Build history of the part. All positions in model axes, mm. A direction names the side the tool comes from. Round coordinates to 2 decimals unless told otherwise and drop trailing zeros. Write each loop counter-clockwise with the first axis right and the second up, starting at its lowest first coordinate (ties: lowest second). Pieces come first, ordered by that corner, then holes. Notation, with made-up numbers: (-11, -26) -> (14, -26) arc R10 cw to (14, -22) -> close; hole circle Ø5 at (78.5, -10.75). An arc over 180 degrees is marked (long way). Answer in a Markdown table with one row per item. Add a question column.
from build123d import *

# Parameters (mm, degrees)
SKETCH1_W           = 20
SKETCH1_H           = 20
BOSS_EXTRUDE1_DEPTH = 10
SKETCH2_R           = 3


with BuildPart() as part:
    # Sketch1 → Boss-Extrude1 (new body)
    with BuildSketch(Plane(origin=(0, 0, 0), x_dir=(1, 0, 0), z_dir=(0, 1, 0))):
        Polygon((-59.044427996, 78.732050808), (-54.714300977, 76.232050808), (-38.661742094, 66.964101615), (-38.661742094, 85.5), (38.661742094, 85.5), (38.661742094, 66.964101615), (54.714300977, 76.232050808), (59.044427996, 78.732050808), (35.218366421, 120), (-35.218366421, 120), align=None)
        with Locations((0, 105)):
            Rectangle(SKETCH1_W, SKETCH1_H, mode=Mode.SUBTRACT)
    extrude(amount=BOSS_EXTRUDE1_DEPTH)

    # Cut-Sweep1: sweep along a path in Sketch3
    with BuildLine(Plane(origin=(0, 5, 0), x_dir=(1, 0, 0), z_dir=(0, 1, 0))) as cut_sweep1_path:
        Line((-38.661742094, 76), (-42.146569651, 76))
        ThreePointArc((-42.146569651, 76), (-43.646569651, 75.598076211), (-44.744645862, 74.5))
        Line((-44.744645862, 74.5), (-46.487059641, 71.482050808))
    # Sketch2 → Cut-Sweep1 (sweep, cut)
    with BuildSketch(Plane(origin=(-38.661742094, 0, 0), x_dir=(0, 0, -1), z_dir=(1, 0, 0))):
        with Locations((76, 5)):
            Circle(SKETCH2_R)
    cut_sweep1 = sweep(path=cut_sweep1_path.line, mode=Mode.SUBTRACT)

    # Mirror3: Cut-Sweep1 across plane
    add(cut_sweep1.mirror(Plane(origin=(0, 0, 0), x_dir=(0, 0, 1), z_dir=(1, 0, 0))), mode=Mode.SUBTRACT)


solid = part.part
(1) Saw through at D-D (z = -98). List the corners of the cut face in (x, y), plus the area to 3 significant figures.
(2) Saw through at A-A (y = 3.5). List the corners of the cut face in (x, z).
(3) Mould opens along Z. For faces 1 (the face through (-1, 5, -85.5)), 2 (the face through (48.106, 4.099, -74.401)), 3 (the face through (47.298, 4.93, -99.077)) say: pulls with the +Z half, pulls with the -Z half, needs draft (parallel to the pull), parting line crosses it, or undercut.
(4) Saw through at C-C (x = 11.5). List the corners of the cut face in (y, z), plus the area to 3 significant figures.
(5) Saw through at B-B (z = -105.5). List the corners of the cut face in (x, y), plus the area to 3 significant figures.
(6) Probe line 1 along Y through (x, z) = (-41.3, -76); line 2 along Z through (x, y) = (-4, 9.5); line 3 along X through (y, z) = (1.5, -77). List the from-to ranges inside material, lowest first.
(7) Which spindle directions (+Z, -Z, +X, -X, +Y, -Y) get a long thin tool onto all of the face, cutting with end or side? Do faces 4 (the face through (40, 5, -73)), 5 (the face through (38.662, 2.7, -78.4)), 6 (the face through (-1, 10, -94)), 7 (the face through (0, 5, -115)). Say none if no direction does.
(8) Drop flat-ended pins along their axis: P1, Ø3.5, axis at y = 5, z = -76, coming from the +X side; P2, Ø1.5, axis at y = 6, z = -91, coming from the -X side; P3, Ø4, axis at y = 8, z = -107, coming from the -X side. Give the stop position or say it passes through.
Answer sheet:
| question | item | result |
|---|---|---|
| 1 | outline | (-47.92, 0) -> (-10, 0) -> (-10, 10) -> (-47.92, 10) -> close; (10, 0) -> (47.92, 0) -> (47.92, 10) -> (10, 10) -> close |
| 1 | area | 758 mm² |
| 2 | outline | (-59.04, -78.73) -> (-35.22, -120) -> (35.22, -120) -> (59.04, -78.73) -> (48.74, -72.78) -> (46.99, -75.8) arc R5.6 cw to (42.15, -78.6) -> (38.66, -78.6) -> (38.66, -85.5) -> (-38.66, -85.5) -> (-38.66, -78.6) -> (-42.15, -78.6) arc R5.6 cw to (-46.99, -75.8) -> (-48.74, -72.78) -> close; (-44.24, -70.18) -> (-42.49, -73.2) arc R0.4 ccw to (-42.15, -73.4) -> (-38.66, -73.4) -> (-38.66, -66.96) -> close; (38.66, -73.4) -> (42.15, -73.4) arc R0.4 ccw to (42.49, -73.2) -> (44.24, -70.18) -> (38.66, -66.96) -> close; hole (-10, -115) -> (10, -115) -> (10, -95) -> (-10, -95) -> close |
| 3 | face 1 | pulls with the +Z half |
| 3 | face 2 | undercut |
| 3 | face 3 | pulls with the -Z half |
| 4 | outline | (0, -120) -> (10, -120) -> (10, -85.5) -> (0, -85.5) -> close |
| 4 | area | 345 mm² |
| 5 | outline | (-43.59, 0) -> (-10, 0) -> (-10, 10) -> (-43.59, 10) -> close; (10, 0) -> (43.59, 0) -> (43.59, 10) -> (10, 10) -> close |
| 5 | area | 672 mm² |
| 6 | line 1 | y = 0 to 2, 8 to 10 |
| 6 | line 2 | z = -120 to -115, -95 to -85.5 |
| 6 | line 3 | x = -56.04 to -38.66, 38.66 to 56.04 |
| 7 | face 4 | none |
| 7 | face 5 | +Z, +Y, -Y |
| 7 | face 6 | +Z, -Z, +X, -X, +Y |
| 7 | face 7 | +Y, -Y |
| 8 | P1 | stops at x = 57.34 |
| 8 | P2 | stops at x = -52.39 |
| 8 | P3 | stops at x = -43.88 |
